from build123d import *

# Parameters (mm, degrees)
F0_R     = 6.6
F2_DEPTH = 16
F3_R     = 10.5
F3_R_2   = 6.6
F4_DEPTH = 4
F5_DEPTH = 15
F6_SIZE  = 5


with BuildPart() as f2:
    # F0 (on Right) → F2 (new body, symmetric)
    with BuildSketch(Plane.YZ):
        with BuildLine():
            Line((31, 13), (0, 13))
            ThreePointArc((0, 13), (-12.489996, 3.605551), (-6.928203, -11))
            Line((-6.928203, -11), (31, -11))
            Line((31, -11), (31, 13))
        make_face()
        Circle(F0_R, mode=Mode.SUBTRACT)
    extrude(amount=F2_DEPTH, both=True)

    # F3 (on face) → F4 (cut)
    with BuildSketch(Plane(origin=(-16, 0, 0), x_dir=(0, -1, 0), z_dir=(-1, 0, 0))):
        Circle(F3_R)
        Circle(F3_R_2, mode=Mode.SUBTRACT)
    extrude(amount=-F4_DEPTH, mode=Mode.SUBTRACT)

    # F1 (on Top) → F5 (cut, symmetric)
    with BuildSketch(Plane.XY):
        with BuildLine():
            Line((-1, -13), (1, -13))
            Line((1, -13), (1, 4.041739))
            ThreePointArc((1, 4.041739), (0, 28), (-1, 4.041739))
            Line((-1, 4.041739), (-1, -13))
        make_face()
    extrude(amount=F5_DEPTH, both=True, mode=Mode.SUBTRACT)

    # F6
    f6_edges = [f2.edges().sort_by_distance(p)[0] for p in [
        (16, 31, 1),
        (-16, 31, 1),
    ]]
    chamfer(f6_edges, length=F6_SIZE)


solid = f2.part
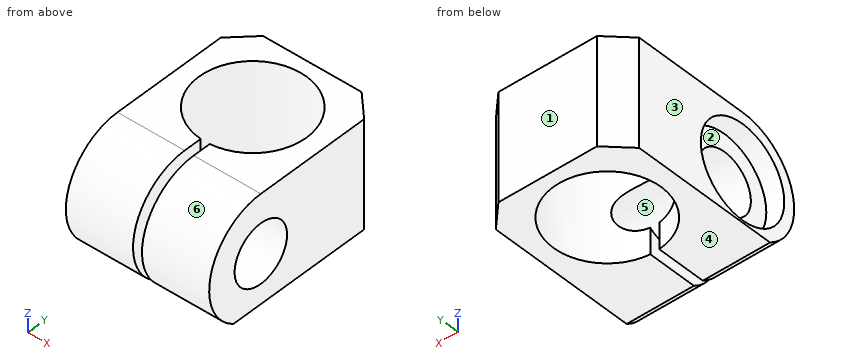
Source: CAD feature listing. Evaluate the final solid. Frame: model axes, mm. Face numbers are marked on the shaded views. A direction names the side the tool comes from. Round coordinates to 2 decimals unless told otherwise and drop trailing zeros. Loops run counter-clockwise (first coordinate to the right, second up) from the corner with the lowest first, then second, coordinate; pieces in that order, holes last. Notation, with made-up numbers: M 70.25,73.5 L 75.25,73.5 A3 ccw 75.25,77.5 Z; hole C -1,71.5 d2. An arc over 180 degrees is marked long. Return JSON: item names as keys, results as strings. Group by question number.
1. Section query C-C on x = -10. Output: boundary loops of the cut face in (y, z), and give its area (3 significant figures).
2. Material intervals for line 1 along Y through (x, z) = (-8, 0); line 2 along X through (y, z) = (3.5, -6.5); line 3 along X through (y, z) = (-10, -3.75), sorted ascending. Write a range as from..to.
3. Section query B-B on x = 6.5. Output: boundary loops of the cut face in (y, z), and give its area (3 significant figures).
4. Section query D-D on z = 0. Output: boundary loops of the cut face in (x, y).
5. Reachability of the marked faces 1 and 2 from +Z, -Z, +X, -X, +Y, -Y: full face, straight path, thin tool, end or side. Return the list, or none.
6. Pin query (flat end, axial travel): pin 1 (6 mm diameter, centred on x = -6, y = 15, fed in from -Z); pin 2 (4 mm diameter, centred on x = 4, y = -1.5, fed in from +Z); pin 3 (5 mm diameter, centred on x = -1.5, z = 3.5, fed in from -Y); pin 4 (10.5 mm diameter, centred on y = -2, z = 2.5, fed in from -X). Return the tip coordinate at first contact, or that it passes through.
7. Section query A-A on y = 16. Output: boundary loops of the cut face in (x, z).
8. Mould query, pull axis Z, two halves, no side actions, for the marked faces 3, 4, 5 and 6. Classes: released by +Z, released by -Z, zero draft, split by the parting line, or undercut.
Checks:
{
 "1": {"outline": "M -6.93,-11 L 9.37,-11 L 9.37,13 L 0,13 A13 ccw Z; M 22.63,-11 L 31,-11 L 31,13 L 22.63,13 Z; hole C 0,0 d13.2", "area": "545 mm²"},
 "2": {"line 1": "y = -13..-6.6, 6.6..7.06, 24.94..31", "line 2": "x = -12..-1, 1..16", "line 3": "x = -16..-1, 1..16"},
 "3": {"outline": "M -6.93,-11 L 5.91,-11 L 5.91,-2.93 A6.6 cw long 5.91,2.93 L 5.91,13 L 0,13 A13 ccw Z; M 26.09,-11 L 31,-11 L 31,13 L 26.09,13 Z", "area": "382 mm²"},
 "4": {"outline": "M -16,-13 L -1,-13 L -1,-6.6 L -12,-6.6 L -12,-10.5 L -16,-10.5 Z; M -16,10.5 L -12,10.5 L -12,6.6 L -7.46,6.6 A12 cw long 7.46,6.6 L 16,6.6 L 16,26 L 11,31 L -11,31 L -16,26 Z; M 1,-13 L 16,-13 L 16,-6.6 L 1,-6.6 Z"},
 "5": {"face 1": "+Z, -Z, +X, -X, +Y", "face 2": "-X"},
 "6": {"pin 1": "passes through", "pin 2": "stops at z = 13", "pin 3": "stops at y = -12.96", "pin 4": "stops at x = -12"},
 "7": {"outline": "M -16,-11 L -12,-11 L -12,13 L -16,13 Z; M 12,-11 L 16,-11 L 16,13 L 12,13 Z"},
 "8": {"face 3": "zero draft", "face 4": "released by -Z", "face 5": "undercut", "face 6": "split by the parting line"}
}
